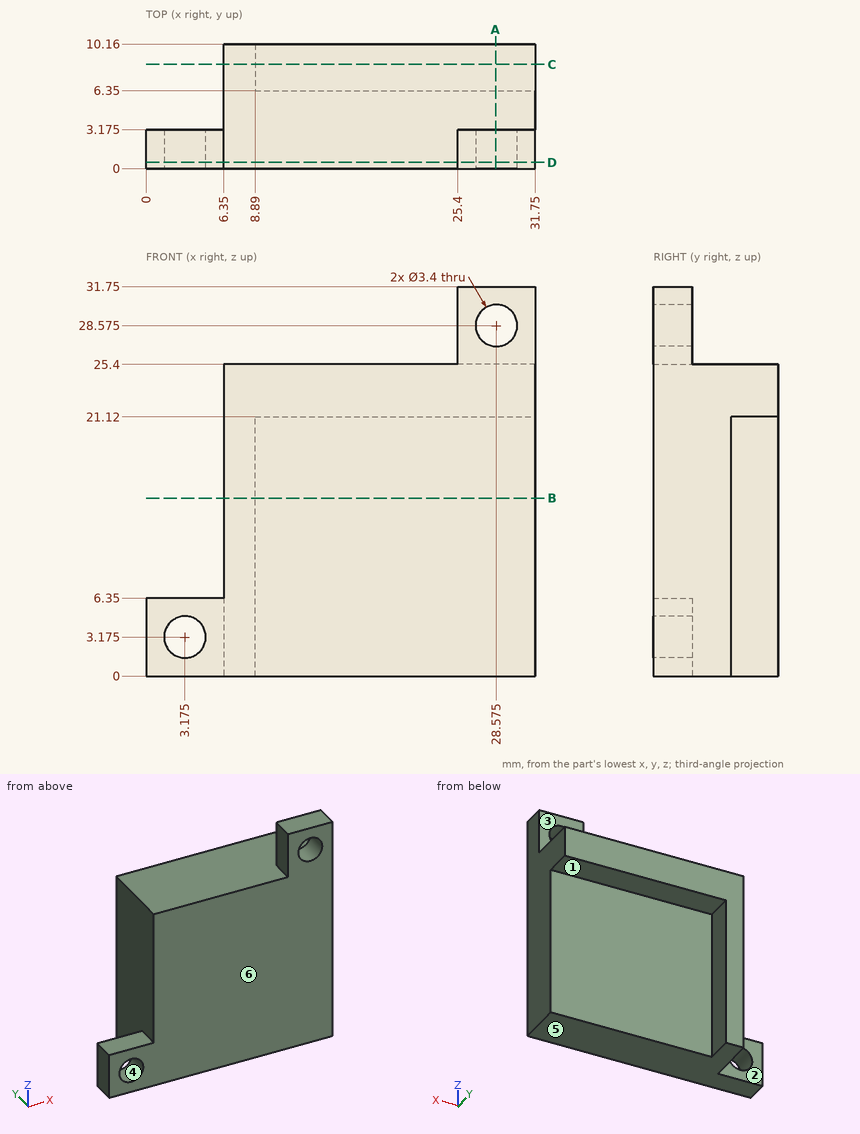
Here's the drawing with two shaded views (mm, measured from the low corner). I have some questions. A direction names the side the tool comes from. Round coordinates to 2 decimals unless told otherwise and drop trailing zeros. Loops run counter-clockwise (first coordinate to the right, second up) from the corner with the lowest first, then second, coordinate; pieces in that order, holes last.
Item 1: Will these pins go through, and if not, where does the flat tip stop? pin 1 Ø3.5 at (y, z) = (2, 29.5) entering from -X; pin 2 Ø1.5 at (x, y) = (18.5, 3.5) entering from +Z; pin 3 Ø1 at (x, y) = (25.5, 7) entering from -Z.
Item 2: Suppose I cut it at D-D, the plane y = 0.5. Write out the boundary of the cut face in (x, z) (3 decimals), then the cut area to 3 significant figures.
Item 3: If we mould it in two halves opening along Z, with no side actions, what happens to the marked faces 4, 5 and 6? For each: +Z half, -Z half, draft (parallel to the pull), parting line (faces both ways), or undercut.
Item 4: Suppose I cut it at B-B, the plane z = 14.5. Write out the boundary of the cut face in (x, y), then the cut area to 3 significant figures.
Item 5: Which directions (+Z, -Z, +X, -X, +Y, -Y) give clear straight access to the entire face, cutting with the end or side of a thin tool? Please do the marked faces 1, 2 and 3.
Item 6: Suppose I cut it at C-C, the plane y = 8.5. Write out the boundary of the cut face in (x, z), then the cut area to 3 significant figures.
Item 7: Suppose I cut it at A-A, the plane x = 28.5. Write out the boundary of the cut face in (y, z) (3 decimals), then the cut area to 3 significant figures.
Item 8: Please list where these lines run through material, in increasing order: L1, parallel to Z at x = 3, y = 2; L2, parallel to Z at x = 20.5, y = 2.5; L3, parallel to Y at x = 5.5, z = 3 (3 decimals).
Reported:
1. pin 1: stops at x = 25.4
1. pin 2: stops at z = 25.4
1. pin 3: stops at z = 21.12
2. outline: (0, 0) - (31.75, 0) - (31.75, 31.75) - (25.4, 31.75) - (25.4, 25.4) - (6.35, 25.4) - (6.35, 6.35) - (0, 6.35) - close; hole circle Ø3.4 at (3.175, 3.175); hole circle Ø3.4 at (28.575, 28.575)
2. area: 708 mm2
3. face 4: undercut
3. face 5: -Z half
3. face 6: draft
4. outline: (6.35, 0) - (31.75, 0) - (31.75, 6.35) - (8.89, 6.35) - (8.89, 10.16) - (6.35, 10.16) - close
4. area: 171 mm2
5. face 1: -Z, +X, +Y
5. face 2: +Z, -Z, -X, +Y
5. face 3: +Z, +X, -X, +Y
6. outline: (6.35, 0) - (8.89, 0) - (8.89, 21.12) - (31.75, 21.12) - (31.75, 25.4) - (6.35, 25.4) - close
6. area: 162 mm2
7. outline: (0, 0) - (6.35, 0) - (6.35, 21.12) - (10.16, 21.12) - (10.16, 25.4) - (3.175, 25.4) - (3.175, 26.877) - (0, 26.877) - close; (0, 30.273) - (3.175, 30.273) - (3.175, 31.75) - (0, 31.75) - close
7. area: 187 mm2
8. L1: z = 0 to 1.48, 4.87 to 6.35
8. L2: z = 0 to 25.4
8. L3: y = 0 to 3.175
